Verification items for this drawing (mm, ordinates from the low corner). Round coordinates to 2 decimals unless told otherwise and drop trailing zeros. Write each loop counter-clockwise with the first axis right and the second up, starting at its lowest first coordinate (ties: lowest second). Pieces come first, ordered by that corner, then holes.
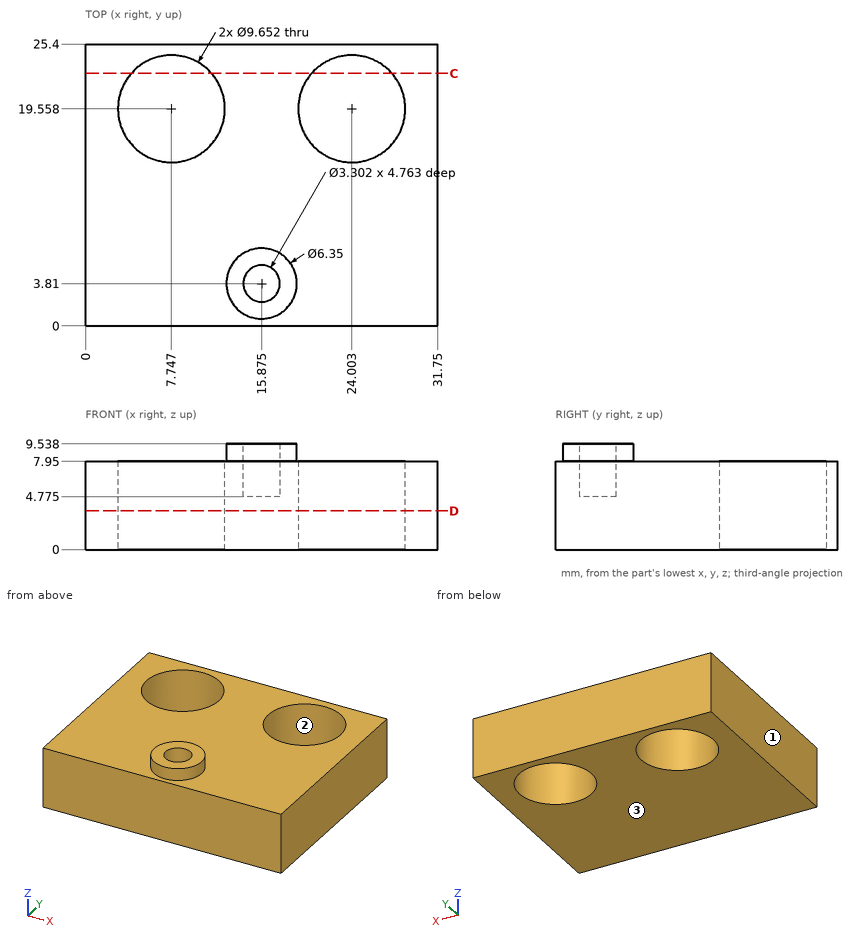
1. Release check for a two-part mould opening along X. For the marked faces 1, 2 and 3 record: +X half, -X half, draft (parallel to the pull), parting line (faces both ways), or undercut.
2. Section check C-C (y = 22.75). Record the cut outline in (x, z).
3. Section check D-D (z = 3.5). State how many separate pieces and enclosed holes the cut face has, plus the area to 3 significant figures.
4. Scan lines: line 1 along X through (y, z) = (17.5, 6); line 2 along Y through (x, z) = (8, 3.25); line 3 along X through (y, z) = (19, 7.25). Record each from-to range of solid material in increasing order.
5. Depth check by flat-ended pin: pin 1 Ø3 at (x, y) = (20.5, 11) entering from +Z. Enter the tip coordinate at first touch or a pass-through.
Results below:
1. face 1: -X half
1. face 2: undercut
1. face 3: draft
2. outline: (0, 0) - (4.13, 0) - (4.13, 7.95) - (0, 7.95) - close; (11.37, 0) - (20.38, 0) - (20.38, 7.95) - (11.37, 7.95) - close; (27.62, 0) - (31.75, 0) - (31.75, 7.95) - (27.62, 7.95) - close
3. separate pieces: 1
3. enclosed holes: 2
3. area: 660 mm2
4. line 1: x = 0 to 3.38, 12.11 to 19.64, 28.37 to 31.75
4. line 2: y = 0 to 14.74, 24.38 to 25.4
4. line 3: x = 0 to 2.95, 12.54 to 19.21, 28.8 to 31.75
5. pin 1: stops at z = 7.95
